Input: part model. Units: mm. Frame: model coordinates. Face numbers are marked on the shaded views. Round coordinates to 2 decimals unless told otherwise and drop trailing zeros. Loops run counter-clockwise (first coordinate to the right, second up) from the corner with the lowest first, then second, coordinate; pieces in that order, holes last.
1) Section A-A, the plane z = 18.5. Return loops of the section in (x, y).
2) Section C-C, the plane z = 5.25. State how many separate pieces and enclosed holes the cut face has, and give its area (3 significant figures).
3) First-contact query: pin 1 (1 mm diameter, centred on x = -5, y = 0, fed in from +Z); pin 2 (1 mm diameter, centred on x = 3.5, y = 0, fed in from +Z); pin 3 (1 mm diameter, centred on y = 0, z = 9.5, fed in from +X). Flat tips, straight axial feed; report the tip coordinate or a pass-through.
4) Draft query along Y for the marked faces 1, 2, 3 and 4. Return one class per face: pulls with the +Y half, pulls with the -Y half, needs draft (parallel to the pull), parting line crosses it, or undercut.
5) Ray query, line 1 along Y through (x, z) = (-3.75, 20.25); line 2 along Y through (x, z) = (-10.5, 14.5); line 3 along Z through (x, y) = (11.5, 1.25). Return the intervals inside material, ascending.
6) Section B-B, the plane x = -10. Return loops of the section in (y, z).
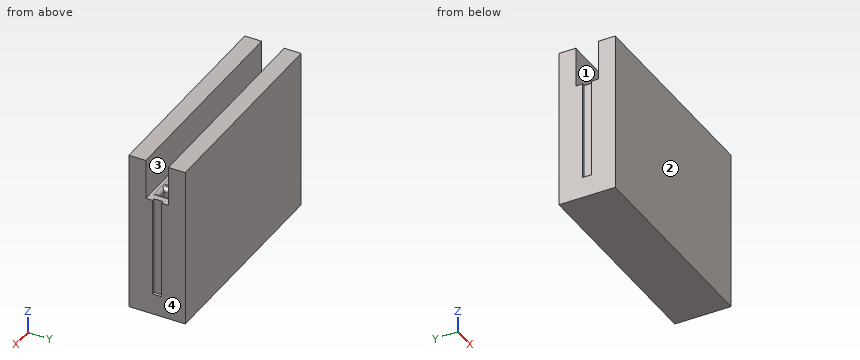
Autodesk Fusion 360 part; units mm, degrees
sketch "Sketch1" plane through (0, 0, 0) normal (0, 0, 1) x (1, 0, 0)
  line L0 (0, 0) -> (15, 0) construction
  line L1 (15, 0) -> (15, 4)
  line L2 (15, 4) -> (0, 4)
  line L3 (0, 4) -> (0, 0) construction
  line L4 (0, 0) -> (0.65, 0) construction
  line L5 (0.65, 0) -> (0.65, 0.65)
  line L6 (0.65, 0.65) -> (0, 0.65)
  line L7 (0, 0.65) -> (0, 0) construction
  line L8 (0.65, -0.65) -> (0, -0.65)
  line L9 (0.65, 0) -> (0.65, -0.65)
  line L10 (-0.65, 0.65) -> (0, 0.65)
  line L11 (-0.65, 0) -> (-0.65, 0.65)
  line L12 (-0.65, 0) -> (-0.65, -0.65)
  line L13 (-0.65, -0.65) -> (0, -0.65)
  line L14 (1.89, 0) -> (1.89, 0.65)
  line L15 (1.89, 0.65) -> (2.54, 0.65)
  line L16 (3.19, 0) -> (3.19, 0.65)
  line L17 (3.19, 0.65) -> (2.54, 0.65)
  line L18 (3.19, 0) -> (3.19, -0.65)
  line L19 (3.19, -0.65) -> (2.54, -0.65)
  line L20 (1.89, 0) -> (1.89, -0.65)
  line L21 (1.89, -0.65) -> (2.54, -0.65)
  line L22 (2.54, 0) -> (17.54, 0) construction
  line L23 (4.43, 0) -> (4.43, 0.65)
  line L24 (4.43, 0.65) -> (5.08, 0.65)
  line L25 (5.73, 0) -> (5.73, 0.65)
  line L26 (5.73, 0.65) -> (5.08, 0.65)
  line L27 (5.73, 0) -> (5.73, -0.65)
  line L28 (5.73, -0.65) -> (5.08, -0.65)
  line L29 (4.43, 0) -> (4.43, -0.65)
  line L30 (4.43, -0.65) -> (5.08, -0.65)
  line L31 (5.08, 0) -> (20.08, 0) construction
  line L32 (6.97, 0) -> (6.97, 0.65)
  line L33 (6.97, 0.65) -> (7.62, 0.65)
  line L34 (8.27, 0) -> (8.27, 0.65)
  line L35 (8.27, 0.65) -> (7.62, 0.65)
  line L36 (8.27, 0) -> (8.27, -0.65)
  line L37 (8.27, -0.65) -> (7.62, -0.65)
  line L38 (6.97, 0) -> (6.97, -0.65)
  line L39 (6.97, -0.65) -> (7.62, -0.65)
  line L40 (7.62, 0) -> (22.62, 0) construction
  line L41 (9.51, 0) -> (9.51, 0.65)
  line L42 (9.51, 0.65) -> (10.16, 0.65)
  line L43 (10.81, 0) -> (10.81, 0.65)
  line L44 (10.81, 0.65) -> (10.16, 0.65)
  line L45 (10.81, 0) -> (10.81, -0.65)
  line L46 (10.81, -0.65) -> (10.16, -0.65)
  line L47 (9.51, 0) -> (9.51, -0.65)
  line L48 (9.51, -0.65) -> (10.16, -0.65)
  line L49 (10.16, 0) -> (25.16, 0) construction
  line L50 (12.05, 0) -> (12.05, 0.65)
  line L51 (12.05, 0.65) -> (12.7, 0.65)
  line L52 (13.35, 0) -> (13.35, 0.65)
  line L53 (13.35, 0.65) -> (12.7, 0.65)
  line L54 (13.35, 0) -> (13.35, -0.65)
  line L55 (13.35, -0.65) -> (12.7, -0.65)
  line L56 (12.05, 0) -> (12.05, -0.65)
  line L57 (12.05, -0.65) -> (12.7, -0.65)
  line L58 (12.7, 0) -> (27.7, 0) construction
  line L59 (14.59, 0) -> (14.59, 0.65)
  line L60 (14.59, 0.65) -> (15.24, 0.65)
  line L61 (15.89, 0) -> (15.89, 0.65)
  line L62 (15.89, 0.65) -> (15.24, 0.65)
  line L63 (15.89, 0) -> (15.89, -0.65)
  line L64 (15.89, -0.65) -> (15.24, -0.65)
  line L65 (14.59, 0) -> (14.59, -0.65)
  line L66 (14.59, -0.65) -> (15.24, -0.65)
  line L67 (15.24, 0) -> (30.24, 0) construction
  line L68 (-3.19, 0) -> (-3.19, 0.65)
  line L69 (-3.19, 0.65) -> (-2.54, 0.65)
  line L70 (-1.89, 0) -> (-1.89, 0.65)
  line L71 (-1.89, 0.65) -> (-2.54, 0.65)
  line L72 (-1.89, 0) -> (-1.89, -0.65)
  line L73 (-1.89, -0.65) -> (-2.54, -0.65)
  line L74 (-3.19, 0) -> (-3.19, -0.65)
  line L75 (-3.19, -0.65) -> (-2.54, -0.65)
  line L76 (-2.54, 0) -> (12.46, 0) construction
  line L77 (-5.73, 0) -> (-5.73, 0.65)
  line L78 (-5.73, 0.65) -> (-5.08, 0.65)
  line L79 (-4.43, 0) -> (-4.43, 0.65)
  line L80 (-4.43, 0.65) -> (-5.08, 0.65)
  line L81 (-4.43, 0) -> (-4.43, -0.65)
  line L82 (-4.43, -0.65) -> (-5.08, -0.65)
  line L83 (-5.73, 0) -> (-5.73, -0.65)
  line L84 (-5.73, -0.65) -> (-5.08, -0.65)
  line L85 (-5.08, 0) -> (9.92, 0) construction
  line L86 (-8.27, 0) -> (-8.27, 0.65)
  line L87 (-8.27, 0.65) -> (-7.62, 0.65)
  line L88 (-6.97, 0) -> (-6.97, 0.65)
  line L89 (-6.97, 0.65) -> (-7.62, 0.65)
  line L90 (-6.97, 0) -> (-6.97, -0.65)
  line L91 (-6.97, -0.65) -> (-7.62, -0.65)
  line L92 (-8.27, 0) -> (-8.27, -0.65)
  line L93 (-8.27, -0.65) -> (-7.62, -0.65)
  line L94 (-7.62, 0) -> (7.38, 0) construction
  line L95 (-10.81, 0) -> (-10.81, 0.65)
  line L96 (-10.81, 0.65) -> (-10.16, 0.65)
  line L97 (-9.51, 0) -> (-9.51, 0.65)
  line L98 (-9.51, 0.65) -> (-10.16, 0.65)
  line L99 (-9.51, 0) -> (-9.51, -0.65)
  line L100 (-9.51, -0.65) -> (-10.16, -0.65)
  line L101 (-10.81, 0) -> (-10.81, -0.65)
  line L102 (-10.81, -0.65) -> (-10.16, -0.65)
  line L103 (-10.16, 0) -> (4.84, 0) construction
  line L104 (-13.35, 0) -> (-13.35, 0.65)
  line L105 (-13.35, 0.65) -> (-12.7, 0.65)
  line L106 (-12.05, 0) -> (-12.05, 0.65)
  line L107 (-12.05, 0.65) -> (-12.7, 0.65)
  line L108 (-12.05, 0) -> (-12.05, -0.65)
  line L109 (-12.05, -0.65) -> (-12.7, -0.65)
  line L110 (-13.35, 0) -> (-13.35, -0.65)
  line L111 (-13.35, -0.65) -> (-12.7, -0.65)
  line L112 (-12.7, 0) -> (2.3, 0) construction
  line L113 (-15.89, 0) -> (-15.89, 0.65)
  line L114 (-15.89, 0.65) -> (-15.24, 0.65)
  line L115 (-14.59, 0) -> (-14.59, 0.65)
  line L116 (-14.59, 0.65) -> (-15.24, 0.65)
  line L117 (-14.59, 0) -> (-14.59, -0.65)
  line L118 (-14.59, -0.65) -> (-15.24, -0.65)
  line L119 (-15.89, 0) -> (-15.89, -0.65)
  line L120 (-15.89, -0.65) -> (-15.24, -0.65)
  line L121 (-15.24, 0) -> (-0.24, 0) construction
  line L122 (15, 0) -> (15, -4)
  line L123 (15, -4) -> (0, -4)
  line L124 (-15, 0) -> (-15, 4)
  line L125 (-15, 4) -> (0, 4)
  line L126 (-15, 0) -> (-15, -4)
  line L127 (-15, -4) -> (0, -4)
  dimension "d1" = 15
  dimension "d2" = 4
  dimension "d3" = 0.65
  dimension "d4" = 0.65
  dimension "d7" = 15.24
  dimension "d8" = 0
  dimension "d11" = -15.24
  dimension "d12" = 0
extrude "Extrude1" add sketch "Sketch1" along normal blind 22.8 contours L1 L2 L59 L60 L65 L66 L115 L116 L117 L118 L122 L123 L124 L125 L126 L127
sketch "Sketch2" plane through (0, 0, 22.8) normal (0, 0, 1) x (-1, 0, 0)
  line L0 (-12.05, 0.65) -> (-12.05, -0.65)
  line L1 (-12.05, -0.65) -> (-13.35, -0.65)
  line L2 (-13.35, -0.65) -> (-13.35, 0.65)
  line L3 (-13.35, 0.65) -> (-12.05, 0.65)
  line L4 (3.19, 0.65) -> (3.19, -0.65)
  line L5 (3.19, -0.65) -> (1.89, -0.65)
  line L6 (1.89, -0.65) -> (1.89, 0.65)
  line L7 (1.89, 0.65) -> (3.19, 0.65)
  line L8 (-9.51, 0.65) -> (-9.51, -0.65)
  line L9 (-9.51, -0.65) -> (-10.81, -0.65)
  line L10 (-10.81, -0.65) -> (-10.81, 0.65)
  line L11 (-10.81, 0.65) -> (-9.51, 0.65)
  line L12 (-6.97, 0.65) -> (-6.97, -0.65)
  line L13 (-6.97, -0.65) -> (-8.27, -0.65)
  line L14 (-8.27, -0.65) -> (-8.27, 0.65)
  line L15 (-8.27, 0.65) -> (-6.97, 0.65)
  line L16 (13.35, 0.65) -> (13.35, -0.65)
  line L17 (13.35, -0.65) -> (12.05, -0.65)
  line L18 (12.05, -0.65) -> (12.05, 0.65)
  line L19 (12.05, 0.65) -> (13.35, 0.65)
  line L20 (8.27, 0.65) -> (8.27, -0.65)
  line L21 (8.27, -0.65) -> (6.97, -0.65)
  line L22 (6.97, -0.65) -> (6.97, 0.65)
  line L23 (6.97, 0.65) -> (8.27, 0.65)
  line L24 (5.73, 0.65) -> (5.73, -0.65)
  line L25 (5.73, -0.65) -> (4.43, -0.65)
  line L26 (4.43, -0.65) -> (4.43, 0.65)
  line L27 (4.43, 0.65) -> (5.73, 0.65)
  line L28 (10.81, 0.65) -> (10.81, -0.65)
  line L29 (10.81, -0.65) -> (9.51, -0.65)
  line L30 (9.51, -0.65) -> (9.51, 0.65)
  line L31 (9.51, 0.65) -> (10.81, 0.65)
  line L32 (-4.43, 0.65) -> (-4.43, -0.65)
  line L33 (-4.43, -0.65) -> (-5.73, -0.65)
  line L34 (-5.73, -0.65) -> (-5.73, 0.65)
  line L35 (-5.73, 0.65) -> (-4.43, 0.65)
  line L36 (-1.89, 0.65) -> (-1.89, -0.65)
  line L37 (-1.89, -0.65) -> (-3.19, -0.65)
  line L38 (-3.19, -0.65) -> (-3.19, 0.65)
  line L39 (-3.19, 0.65) -> (-1.89, 0.65)
  line L40 (0.65, 0.65) -> (0.65, -0.65)
  line L41 (0.65, -0.65) -> (-0.65, -0.65)
  line L42 (-0.65, -0.65) -> (-0.65, 0.65)
  line L43 (-0.65, 0.65) -> (0.65, 0.65)
  line L44 (14.59, -0.65) -> (14.59, 0.65)
  line L45 (14.59, 0.65) -> (15, 0.65)
  line L46 (15, 0.65) -> (15, 4)
  line L47 (15, 4) -> (-15, 4)
  line L48 (-15, 4) -> (-15, 0.65)
  line L49 (-15, 0.65) -> (-14.59, 0.65)
  line L50 (-14.59, 0.65) -> (-14.59, -0.65)
  line L51 (-14.59, -0.65) -> (-15, -0.65)
  line L52 (-15, -0.65) -> (-15, -4)
  line L53 (-15, -4) -> (15, -4)
  line L54 (15, -4) -> (15, -0.65)
  line L55 (15, -0.65) -> (14.59, -0.65)
  line L56 (0, 0) -> (-15, 0) construction
  line L57 (-15, 0) -> (-15, -1.6)
  line L58 (-15, -1.6) -> (0, -1.6)
  line L59 (0, -1.6) -> (0, 0) construction
  line L60 (-15, 0) -> (-15, 1.6)
  line L61 (-15, 1.6) -> (0, 1.6)
  line L62 (15, 0) -> (15, -1.6)
  line L63 (15, -1.6) -> (0, -1.6)
  line L64 (15, 0) -> (15, 1.6)
  line L65 (15, 1.6) -> (0, 1.6)
  dimension "d15" = 1.6
extrude "Extrude2" cut sketch "Sketch2" against normal blind 5.7 contours L44 L45 L46 L48 L49 L50 L51 L52 L54 L55 L57 L58 L60 L61 L62 L63 L64 L65
extrude "Extrude4" add sketch "Sketch1" along normal blind 3 contours L1 L59 L60 L65 L66 L122 | L1 L2 L59 L60 L65 L66 L115 L116 L117 L118 L122 L123 L124 L125 L126 L127 | L115 L116 L117 L118 L124 L126 | L5 L6 L8 L9 L10 L11 L12 L13 | L14 L15 L16 L17 L18 L19 L20 L21 | L23 L24 L25 L26 L27 L28 L29 L30 | L32 L33 L34 L35 L36 L37 L38 L39 | L41 L42 L43 L44 L45 L46 L47 L48 | L50 L51 L52 L53 L54 L55 L56 L57 | L68 L69 L70 L71 L72 L73 L74 L75 | L77 L78 L79 L80 L81 L82 L83 L84 | L86 L87 L88 L89 L90 L91 L92 L93 | L95 L96 L97 L98 L99 L100 L101 L102 | L104 L105 L106 L107 L108 L109 L110 L111
fillet "Fillet1" radius 0.5 44 edges at (-13.35, 0, 17.1) (-12.7, 0.65, 17.1) (-12.05, 0, 17.1) (-12.7, -0.65, 17.1) (-10.81, 0, 17.1) (-10.16, 0.65, 17.1) (-10.16, -0.65, 17.1) (-9.51, 0, 17.1) (-8.27, 0, 17.1) (-7.62, 0.65, 17.1) (-6.97, 0, 17.1) (-7.62, -0.65, 17.1) (-5.73, 0, 17.1) (-5.08, 0.65, 17.1) (-4.43, 0, 17.1) (-5.08, -0.65, 17.1) (-3.19, 0, 17.1) (-2.54, 0.65, 17.1) (-1.89, 0, 17.1) (-2.54, -0.65, 17.1) (-0.65, 0, 17.1) (0, 0.65, 17.1) (0.65, 0, 17.1) (0, -0.65, 17.1) (1.89, 0, 17.1) (2.54, 0.65, 17.1) (3.19, 0, 17.1) (2.54, -0.65, 17.1) (4.43, 0, 17.1) (5.08, 0.65, 17.1) (5.73, 0, 17.1) (5.08, -0.65, 17.1) (6.97, 0, 17.1) (7.62, 0.65, 17.1) (8.27, 0, 17.1) (7.62, -0.65, 17.1) (9.51, 0, 17.1) (10.16, 0.65, 17.1) (10.81, 0, 17.1) (10.16, -0.65, 17.1) (12.05, 0, 17.1) (12.7, 0.65, 17.1) (13.35, 0, 17.1) (12.7, -0.65, 17.1)
equation "d3 = d4"
Final values:
1. outline: (-15, -4) - (15, -4) - (15, -1.6) - (-15, -1.6) - close; (-15, 1.6) - (15, 1.6) - (15, 4) - (-15, 4) - close
2. separate pieces: 1
2. enclosed holes: 11
2. area: 220 mm2
3. pin 1: stops at z = 3
3. pin 2: stops at z = 17.1
3. pin 3: stops at x = 14.59
4. face 1: undercut
4. face 2: pulls with the -Y half
4. face 3: undercut
4. face 4: needs draft
5. line 1: y = -4 to -1.6, 1.6 to 4
5. line 2: y = -4 to -0.65, 0.65 to 4
5. line 3: z = 0 to 17.1
6. outline: (-4, 0) - (4, 0) - (4, 22.8) - (1.6, 22.8) - (1.6, 17.1) - (1.15, 17.1) arc R0.5 ccw to (0.65, 16.6) - (0.65, 3) - (-0.65, 3) - (-0.65, 16.6) arc R0.5 ccw to (-1.15, 17.1) - (-1.6, 17.1) - (-1.6, 22.8) - (-4, 22.8) - close
